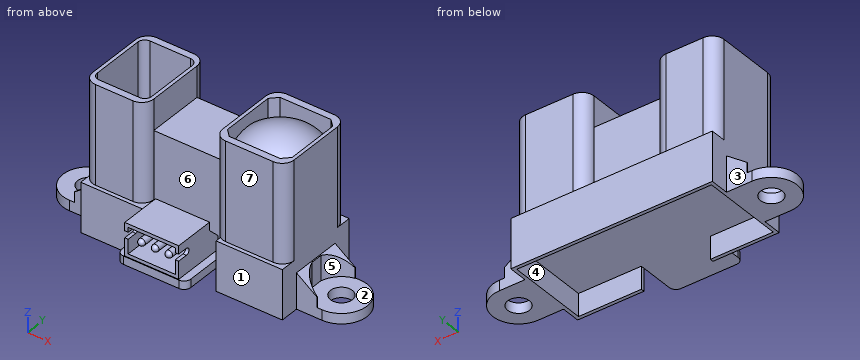
from build123d import *

# Parameters (mm, degrees)
SKETCH1_R                = 1.6
BOSS_EXTRUDE1_DEPTH      = 7.2
CUT_EXTRUDE1_DEPTH       = 46.901288027
CUT_EXTRUDE2_DEPTH       = 45.728108035
BOSS_EXTRUDE4_DEPTH      = 14.4
SKETCH6_W                = 10.1
SKETCH6_H                = 8.4
BOSS_EXTRUDE5_DEPTH      = 9.9
REVOLVE1_ANGLE           = 180
CUT_EXTRUDE3_DEPTH       = 4
SKETCH13_W               = 28.5
SKETCH13_H               = 12
CUT_EXTRUDE4_DEPTH       = 3.3
BOSS_EXTRUDE6_DEPTH      = 1.2
BOSS_EXTRUDE7_DEPTH      = 3.95
BOSS_EXTRUDE7_DEPTH_BACK = 3.95
SKETCH16_W               = 6.9
SKETCH16_H               = 3.8
CUT_EXTRUDE5_DEPTH       = 5.5
SKETCH18_R               = 0.5
BOSS_EXTRUDE8_DEPTH      = 5.25
FILLET1_R                = 0.5


with BuildPart() as part:
    # Sketch1 → Boss-Extrude1 (new body)
    with BuildSketch(Plane.XY):
        with BuildLine():
            Line((-39.67911745, 6.306787833), (-35.92911745, 6.306787833))
            Line((-35.92911745, 6.306787833), (-35.92911745, 9.056787833))
            Line((-35.92911745, 9.056787833), (-6.42911745, 9.056787833))
            Line((-6.42911745, 9.056787833), (-6.42911745, 6.306787833))
            Line((-6.42911745, 6.306787833), (-2.67911745, 6.306787833))
            ThreePointArc((-2.67911745, 6.306787833), (1.07088255, 2.556787833), (-2.67911745, -1.193212167))
            Line((-2.67911745, -1.193212167), (-6.42911745, -1.193212167))
            Line((-6.42911745, -1.193212167), (-6.42911745, -3.943212167))
            Line((-6.42911745, -3.943212167), (-16.12911745, -3.943212167))
            Line((-16.12911745, -3.943212167), (-16.12911745, -3.079352829))
            ThreePointArc((-16.12911745, -3.079352829), (-16.680326656, -2.453304755), (-16.87911745, -1.643212167))
            Line((-16.87911745, -1.643212167), (-25.47911745, -1.643212167))
            ThreePointArc((-25.47911745, -1.643212167), (-25.677908244, -2.453304755), (-26.22911745, -3.079352829))
            Line((-26.22911745, -3.079352829), (-26.22911745, -3.943212167))
            Line((-26.22911745, -3.943212167), (-35.92911745, -3.943212167))
            Line((-35.92911745, -3.943212167), (-35.92911745, -1.193212167))
            Line((-35.92911745, -1.193212167), (-39.67911745, -1.193212167))
            ThreePointArc((-39.67911745, -1.193212167), (-43.42911745, 2.556787833), (-39.67911745, 6.306787833))
        make_face()
        with Locations((-39.67911745, 2.556787833)):
            Circle(SKETCH1_R, mode=Mode.SUBTRACT)
        with Locations((-2.67911745, 2.556787833)):
            Circle(SKETCH1_R, mode=Mode.SUBTRACT)
    extrude(amount=BOSS_EXTRUDE1_DEPTH)

    # Sketch3 → Cut-Extrude1 (cut, through all)
    with BuildSketch(Plane.XZ.offset(3.943212167)):
        Polygon((-44.543539252, 1.5), (-38.92911745, 1.5), (-38.92911745, 3), (-35.92911745, 5.2), (-35.92911745, 8.378943839), (-44.543539252, 8.378943839), align=None)
        Polygon((2.185304351, 8.378943839), (2.185304351, 1.5), (-3.42911745, 1.5), (-3.42911745, 3), (-6.42911745, 5.2), (-6.42911745, 8.378943839), align=None)
    extrude(amount=-CUT_EXTRUDE1_DEPTH, mode=Mode.SUBTRACT)

    # Sketch4 → Cut-Extrude2 (cut, through all)
    with BuildSketch(Plane.XY.offset(1.5)):
        with BuildLine():
            Line((-36.02911745, 3.417020359), (-36.02911745, 1.696555306))
            ThreePointArc((-36.02911745, 1.696555306), (-43.42911745, 2.556787833), (-36.02911745, 3.417020359))
        make_face()
        with BuildLine():
            Line((-6.32911745, 3.417020359), (-6.32911745, 1.696555306))
            ThreePointArc((-6.32911745, 1.696555306), (1.07088255, 2.556787833), (-6.32911745, 3.417020359))
        make_face()
    extrude(amount=CUT_EXTRUDE2_DEPTH, mode=Mode.SUBTRACT)

    # Sketch5 → Boss-Extrude4 (add)
    # profile 1 of 2: a face of its own
    with BuildSketch(Plane.XY.offset(7.2)):
        with BuildLine():
            Line((-34.17911745, 8.506787833), (-28.72911745, 8.506787833))
            ThreePointArc((-28.72911745, 8.506787833), (-27.491680583, 7.9942247), (-26.97911745, 6.756787833))
            Line((-26.97911745, 6.756787833), (-26.97911745, -1.643212167))
            ThreePointArc((-26.97911745, -1.643212167), (-27.491680583, -2.880649034), (-28.72911745, -3.393212167))
            Line((-28.72911745, -3.393212167), (-34.17911745, -3.393212167))
            ThreePointArc((-34.17911745, -3.393212167), (-35.416554317, -2.880649034), (-35.92911745, -1.643212167))
            Line((-35.92911745, -1.643212167), (-35.92911745, 6.756787833))
            ThreePointArc((-35.92911745, 6.756787833), (-35.416554317, 7.9942247), (-34.17911745, 8.506787833))
        make_face()
        with BuildLine():
            Line((-34.42911745, 7.506787833), (-28.47911745, 7.506787833))
            ThreePointArc((-28.47911745, 7.506787833), (-27.772010669, 7.213894614), (-27.47911745, 6.506787833))
            Line((-27.47911745, 6.506787833), (-27.47911745, -1.393212167))
            ThreePointArc((-27.47911745, -1.393212167), (-27.772010669, -2.100318948), (-28.47911745, -2.393212167))
            Line((-28.47911745, -2.393212167), (-34.42911745, -2.393212167))
            ThreePointArc((-34.42911745, -2.393212167), (-35.136224231, -2.100318948), (-35.42911745, -1.393212167))
            Line((-35.42911745, -1.393212167), (-35.42911745, 6.506787833))
            ThreePointArc((-35.42911745, 6.506787833), (-35.136224231, 7.213894614), (-34.42911745, 7.506787833))
        make_face(mode=Mode.SUBTRACT)
    # profile 2 of 2: a face of its own
    with BuildSketch(Plane.XY.offset(7.2)):
        with BuildLine():
            Line((-15.12911745, 8.506787833), (-8.17911745, 8.506787833))
            ThreePointArc((-8.17911745, 8.506787833), (-6.941680583, 7.9942247), (-6.42911745, 6.756787833))
            Line((-6.42911745, 6.756787833), (-6.42911745, -1.643212167))
            ThreePointArc((-6.42911745, -1.643212167), (-6.941680583, -2.880649034), (-8.17911745, -3.393212167))
            Line((-8.17911745, -3.393212167), (-15.12911745, -3.393212167))
            ThreePointArc((-15.12911745, -3.393212167), (-16.366554317, -2.880649034), (-16.87911745, -1.643212167))
            Line((-16.87911745, -1.643212167), (-16.87911745, 6.756787833))
            ThreePointArc((-16.87911745, 6.756787833), (-16.366554317, 7.9942247), (-15.12911745, 8.506787833))
        make_face()
        Polygon((-15.37911745, 7.506787833), (-7.92911745, 7.506787833), (-6.92911745, 6.506787833), (-6.92911745, -1.393212167), (-7.92911745, -2.393212167), (-15.37911745, -2.393212167), (-16.37911745, -1.393212167), (-16.37911745, 6.506787833), align=None, mode=Mode.SUBTRACT)
    extrude(amount=BOSS_EXTRUDE4_DEPTH)

    # Sketch6 → Boss-Extrude5 (add)
    with BuildSketch(Plane.XY.offset(7.2)):
        with Locations((-21.92911745, 2.556787833)):
            Rectangle(SKETCH6_W, SKETCH6_H)
    extrude(amount=BOSS_EXTRUDE5_DEPTH)

    # Sketch7 → Revolve1 (revolve)
    with BuildSketch(Plane.XY.offset(7.2)):
        with BuildLine():
            Line((-31.45411745, 6.527394978), (-31.45411745, -1.272605022))
            ThreePointArc((-31.45411745, -1.272605022), (-27.55411745, 2.627394978), (-31.45411745, 6.527394978))
        make_face()
    revolve(axis=Axis((-31.45411745, 8.506787833, 7.2), (0, -1, 0)), revolution_arc=REVOLVE1_ANGLE)

    # Sketch11 → Revolve7 (revolve)
    with BuildSketch(Plane(origin=(-11.65411745, 0, 0), x_dir=(0, 0, -1), z_dir=(1, 0, 0))):
        with BuildLine():
            Line((-17.85, 9.006787833), (-17.85, 2.556787833))
            Line((-17.85, 2.556787833), (-21.522794753, 2.556787833))
            ThreePointArc((-21.522794753, 2.556787833), (-20.54023441, 6.267984449), (-17.85, 9.006787833))
        make_face()
    revolve(axis=Axis((-11.65411745, 2.556787833, 6.48), (0, 0, 1)))

    # Sketch12 → Cut-Extrude3 (cut)
    with BuildSketch(Plane.XY.offset(21.6)):
        with BuildLine():
            Line((-9.164137531, 8.506787833), (-14.14409737, 8.506787833))
            ThreePointArc((-14.14409737, 8.506787833), (-11.65411745, 9.006787833), (-9.164137531, 8.506787833))
        make_face()
        with BuildLine():
            Line((-6.42911745, -1.224994155), (-6.42911745, 6.33856982))
            ThreePointArc((-6.42911745, 6.33856982), (-5.20411745, 2.556787833), (-6.42911745, -1.224994155))
        make_face()
        with BuildLine():
            Line((-14.14409737, -3.393212167), (-9.164137531, -3.393212167))
            ThreePointArc((-9.164137531, -3.393212167), (-11.65411745, -3.893212167), (-14.14409737, -3.393212167))
        make_face()
        with BuildLine():
            Line((-16.87911745, 6.33856982), (-16.87911745, -1.224994155))
            ThreePointArc((-16.87911745, -1.224994155), (-18.10411745, 2.556787833), (-16.87911745, 6.33856982))
        make_face()
    extrude(amount=-CUT_EXTRUDE3_DEPTH, mode=Mode.SUBTRACT)

    # Sketch13 → Cut-Extrude4 (cut)
    with BuildSketch(Plane(origin=(0, 0, 0), x_dir=(-1, 0, 0), z_dir=(0, 0, -1))):
        with Locations((21.17911745, 2.556787833)):
            Rectangle(SKETCH13_W, SKETCH13_H)
    extrude(amount=-CUT_EXTRUDE4_DEPTH, mode=Mode.SUBTRACT)

    # Sketch14 → Boss-Extrude6 (add)
    with BuildSketch(Plane(origin=(0, 0, 3.3), x_dir=(-1, 0, 0), z_dir=(0, 0, -1))):
        with BuildLine():
            Line((26.22911745, -3.943212167), (26.22911745, -3.079352829))
            ThreePointArc((26.22911745, -3.079352829), (25.677908244, -2.453304755), (25.47911745, -1.643212167))
            Line((25.47911745, -1.643212167), (16.87911745, -1.643212167))
            ThreePointArc((16.87911745, -1.643212167), (16.680326656, -2.453304755), (16.12911745, -3.079352829))
            Line((16.12911745, -3.079352829), (16.12911745, -3.943212167))
            Line((16.12911745, -3.943212167), (16.12911745, -8.843212167))
            ThreePointArc((16.12911745, -8.843212167), (16.422010669, -9.550318948), (17.12911745, -9.843212167))
            Line((17.12911745, -9.843212167), (25.22911745, -9.843212167))
            ThreePointArc((25.22911745, -9.843212167), (25.936224231, -9.550318948), (26.22911745, -8.843212167))
            Line((26.22911745, -8.843212167), (26.22911745, -3.943212167))
        make_face()
    extrude(amount=-BOSS_EXTRUDE6_DEPTH)

    # Sketch15 → Boss-Extrude7 (add, two sides: drawn at the far end of the back side and taken through both)
    with BuildSketch(Plane.ZY.offset(21.17911745).offset(-BOSS_EXTRUDE7_DEPTH_BACK)):
        with BuildLine():
            Line((6.5, -2.143212167), (4.5, -2.143212167))
            Line((4.5, -2.143212167), (4.5, -9.743212167))
            Line((4.5, -9.743212167), (7.1, -9.743212167))
            Line((7.1, -9.743212167), (7.1, -8.243212167))
            ThreePointArc((7.1, -8.243212167), (7.6, -7.743212167), (8.1, -8.243212167))
            Line((8.1, -8.243212167), (8.1, -9.743212167))
            Line((8.1, -9.743212167), (9.3, -9.743212167))
            Line((9.3, -9.743212167), (9.3, -3.743212167))
            Line((9.3, -3.743212167), (8.1, -3.743212167))
            Line((8.1, -3.743212167), (6.5, -2.143212167))
        make_face()
    extrude(amount=BOSS_EXTRUDE7_DEPTH + BOSS_EXTRUDE7_DEPTH_BACK)

    # Sketch16 → Cut-Extrude5 (cut)
    with BuildSketch(Plane.XZ.offset(9.743212167)):
        with Locations((-21.17911745, 6.9)):
            Rectangle(SKETCH16_W, SKETCH16_H)
    extrude(amount=-CUT_EXTRUDE5_DEPTH, mode=Mode.SUBTRACT)

    # Sketch18 → Boss-Extrude8 (add)
    with BuildSketch(Plane.XZ.offset(4.243212167)):
        with Locations(Location((-21.17911745, 6.9, 0), (0, 0, 270))):
            Circle(SKETCH18_R)
        with Locations(Location((-19.17911745, 6.9, 0), (0, 0, 270))):
            Circle(SKETCH18_R)
        with Locations(Location((-23.17911745, 6.9, 0), (0, 0, 270))):
            Circle(SKETCH18_R)
    extrude(amount=BOSS_EXTRUDE8_DEPTH)

    # Fillet1
    fillet1_edges = [part.edges().sort_by_distance(p)[0] for p in [
        (-21.17911745, -9.493212167, 7.4),
        (-19.17911745, -9.493212167, 7.4),
        (-23.17911745, -9.493212167, 7.4),
    ]]
    fillet(fillet1_edges, radius=FILLET1_R)


solid = part.part
The model under review builds one solid part; all positions refer to its coordinate system, in mm. Face numbers are marked on the shaded views. A direction names the side the tool comes from. Coordinates: 2 decimals unless noted, no trailing zeros. Write each loop counter-clockwise with the first axis right and the second up, starting at its lowest first coordinate (ties: lowest second). Pieces come first, ordered by that corner, then holes. Notation, with made-up numbers: M 52.5,-13.75 L 99.5,-13.75 A33 ccw 99.5,23.25 Z; hole C 60,18 d1. An arc over 180 degrees is marked long. Put each result on its own line as item: value.
1) Add section B-B on z = 15.75. State how many separate pieces and enclosed holes the cut face has, then the cut area to 3 significant figures.
Computed:
separate pieces: 1
enclosed holes: 2
area: 141 mm2
2) Clearance check with flat-ended pins moving along their axes: pin 1 Ø4 at (y, z) = (-1, 8.5) entering from -X; pin 2 Ø1.3 at (y, z) = (4, 19.5) entering from +X; pin 3 Ø1.9 at (x, y) = (-2.68, 2.56) entering from +Z; pin 4 Ø1.8 at (x, z) = (-31, 17.5) entering from +Y. State where each tip first meets the part, or that it passes through.
Computed:
pin 1: stops at x = -35.93
pin 2: stops at x = -6.43
pin 3: passes through
pin 4: stops at y = 8.51
3) Draft analysis for pull direction X (two halves, no side actions). For the marked faces 4, 5, 6 and 7, state which applies: released by +X, released by -X, zero draft, split by the parting line, or undercut.
Computed:
face 4: undercut
face 5: released by +X
face 6: undercut
face 7: zero draft
4) For the marked faces 1, 2 and 3, list the 3-axis set-ups (+Z, -Z, +X, -X, +Y, -Y) from which the entire face can be reached by the end or side of a thin tool; tool diameter is ignored.
Computed:
face 1: +Z, -Z, +X, -Y
face 2: +Z, +X
face 3: +Z, -Z, -X, +Y
5) Add section D-D on x = -12.5. Give the boundary of the cut face in (y, z).
Computed:
outline: M -3.94,0 L -3.44,0 L -3.44,3.3 L 8.56,3.3 L 8.56,0 L 9.06,0 L 9.06,7.2 L 8.51,7.2 L 8.51,21.6 L 7.51,21.6 L 7.51,19.59 A7.45 ccw -2.39,19.59 L -2.39,21.6 L -3.39,21.6 L -3.39,7.2 L -3.94,7.2 Z; hole M -2.39,7.2 L 7.51,7.2 L 7.51,17.85 L -2.39,17.85 Z
6) Add section A-A on y = -6.5. Give the boundary of the cut face in (x, z), then the cut area to 3 significant figures.
Computed:
outline: M -26.23,3.3 L -16.13,3.3 L -16.13,4.5 L -17.23,4.5 L -17.23,9.3 L -25.13,9.3 L -25.13,4.5 L -26.23,4.5 Z; C -23.18,6.9 d1; C -21.18,6.9 d1; C -19.18,6.9 d1; hole M -24.63,5 L -17.73,5 L -17.73,8.8 L -24.63,8.8 Z
area: 26.2 mm2
7) Wall thickness on probe 1 along X at (y, z) = (0, 13.5); probe 2 along X at (y, z) = (2.5, 19.5); probe 3 along Y at (x, z) = (-19.5, 8.5): over which ranges is each line inside the solid? List them lowest first. Write a range as [from, to].
Computed:
probe 1: x = [-35.93, -35.43], [-27.48, -16.38], [-6.93, -6.43]
probe 2: x = [-35.93, -35.43], [-27.48, -26.98], [-16.88, -6.43]
probe 3: y = [-4.24, -3.74], [-1.64, 6.76]
